The drawing under review shows one solid part. Ordinate dimensions are in mm from its lowest x, y, z. A direction names the side the tool comes from. Coordinates: 2 decimals unless noted, no trailing zeros. Loops run counter-clockwise (first coordinate to the right, second up) from the corner with the lowest first, then second, coordinate; pieces in that order, holes last. Notation, with made-up numbers: M -20.75,18 L 33.25,18 A6 ccw 33.25,26 Z; hole C -21.5,-28 d10. An arc over 180 degrees is marked long. Use one line per item in the form item = value.
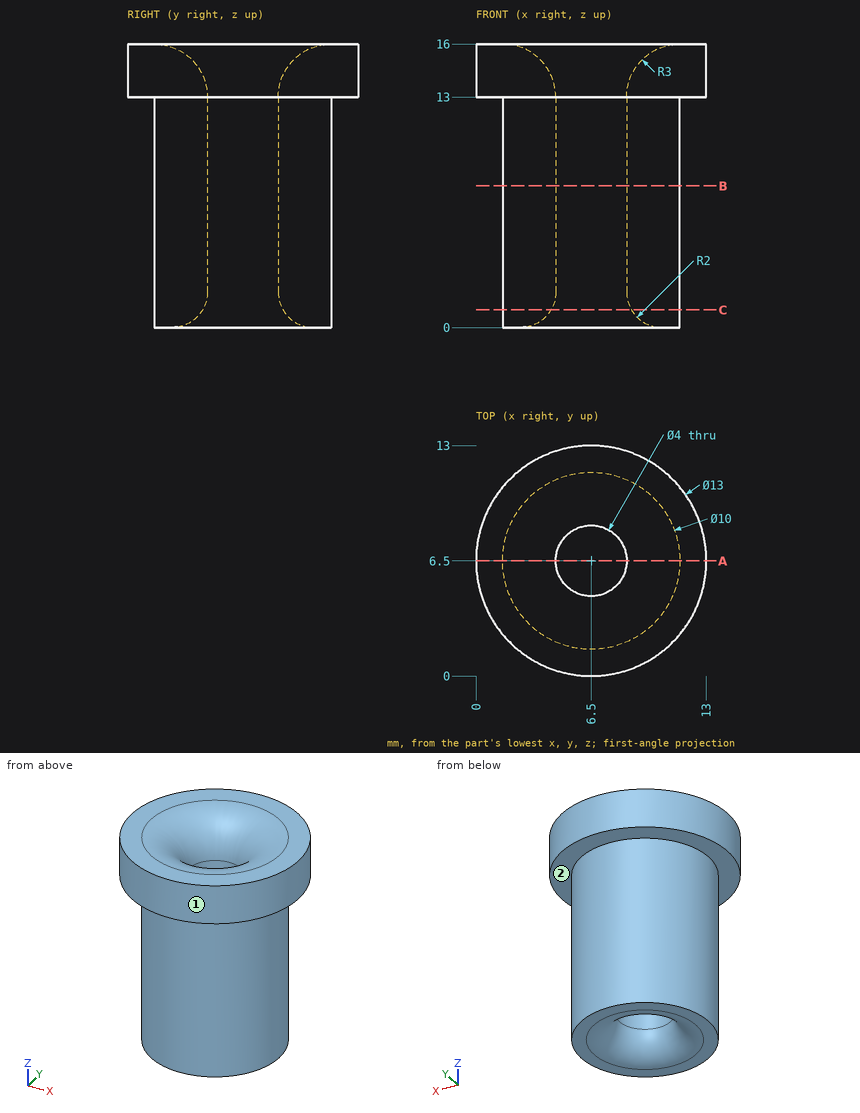
1. For pin 1 Ø1.5 at (x, z) = (4.5, 13) entering from -Y; pin 2 Ø4 at (y, z) = (5.5, 4) entering from -X, all flat-tipped, find the tip position at first contact; note any pin that passes through.
Computed values:
pin_1 = 0.12
pin_2 = 1.5
2. Wall thickness on line 1 along X through (y, z) = (6.5, 9.75); line 2 along Z through (x, y) = (2, 8.5): over which ranges is each line inside the solid? List them lowest first. Write a range as from..to.
Computed values:
line_1 = 1.5..4.5, 8.5..11.5
line_2 = 0..16
3. Consider section B-B on z = 8. Write out the cut boundary in (x, y), plus the area to 3 significant figures.
Computed values:
outline = C 6.5,6.5 d10; hole C 6.5,6.5 d4
area = 66.0 mm2
4. Consider section C-C on z = 1. Write out the cut boundary in (x, y).
Computed values:
outline = C 6.5,6.5 d10; hole C 6.5,6.5 d4.54
5. Tool access review of the marked faces 1 and 2: name each direction out of +Z, -Z, +X, -X, +Y, -Y from which nothing blocks a thin tool from reaching the whole face with its end or side.
Computed values:
face_1 = +Z, -Z
face_2 = -Z
6. Consider section A-A on y = 6.5. Write out the cut boundary in (x, z), plus the area to 3 significant figures.
Computed values:
outline = M 0,13 L 1.5,13 L 1.5,0 L 2.5,0 A2 ccw 4.5,2 L 4.5,13 A3 ccw 1.5,16 L 0,16 Z; M 8.5,2 A2 ccw 10.5,0 L 11.5,0 L 11.5,13 L 13,13 L 13,16 L 11.5,16 A3 ccw 8.5,13 Z
area = 99.4 mm2
